Could you check a few things on this model? Use its own coordinates, in mm. A direction names the side the tool comes from. Coordinates: 2 decimals unless noted, no trailing zeros. Write each loop counter-clockwise with the first axis right and the second up, starting at its lowest first coordinate (ties: lowest second). Pieces come first, ordered by that corner, then holes.
Item 1: If I drill on probe 1 along Y at (x, z) = (2, -11.5); probe 2 along X at (y, z) = (45, -7.25); probe 3 along Y at (x, z) = (3, -6.5), over which ranges is the centre line in solid material (lowest first)?
Item 2: I want a section at C-C on x = 13. Please give me the cut outline in (y, z).
Item 3: I want a section at B-B on y = 51.5. Please give me the cut outline in (x, z).
Item 4: Which directions (+Z, -Z, +X, -X, +Y, -Y) give clear straight access to the entire face, cutting with the end or side of a thin tool? Please do faces 5 (the flat face through (9, 153.67, -4)), 6 (the flat face through (1, 0, -2)), 7 (the flat face through (-11, 0, -12)).
Item 5: I want a section at A-A on x = -9.5. Please give me the cut outline in (y, z).
Item 6: For P1, Ø1.5, axis at x = 4.5, y = 38, coming from the -Z side; P2, Ø0.6, axis at x = 1.5, z = -11.5, coming from the -Y side; P3, Ø1, axis at y = 22, z = -2.5, coming from the -X side; P4, Ø1.5, axis at y = 115.5, z = -6, coming from the +X side, each with a flat end and sliding along its axis, tell me the tip position at first contact or that it passes through.
Item 7: Thinking about a two-plate mould opening in X: for faces 1 (the flat face through (2.172, 77, -4)), 2 (the flat face through (9, 152.4, -4)), 3 (the flat face through (-0.876, 76, -4)), 4 (the flat face through (1, 0, -7)), which applies, +X half, -X half, draft (parallel to the pull), parting line (faces both ways), or undercut?
from build123d import *

# Parameters (mm, degrees)
BOSS_EXTRUDE1_DEPTH = 152.4
SKETCH2_W           = 19.05
SKETCH2_H           = 19.05
BOSS_EXTRUDE2_DEPTH = 1.27
SKETCH3_R           = 1.016
BOSS_EXTRUDE3_DEPTH = 8.89
BOSS_EXTRUDE4_DEPTH = 1.27
SKETCH5_W           = 15.24
SKETCH5_H           = 12.7
CUT_EXTRUDE1_DEPTH  = 2.27


with BuildPart() as part:
    # Sketch1 → Boss-Extrude1 (new body)
    with BuildSketch(Plane(origin=(0, 0, 0), x_dir=(1, 0, 0), z_dir=(0, 1, 0))):
        Polygon((0.1397, 7.023481), (-0.8763, 7.023481), (-0.8763, 1.305306), (0.1397, 1.305306), (0.1397, 0), (2.1717, 0), (2.1717, 8.328787), (0.1397, 8.328787), align=None)
    extrude(amount=BOSS_EXTRUDE1_DEPTH)

    # Sketch2 → Boss-Extrude2 (add)
    with BuildSketch(Plane(origin=(0, 152.4, 0), x_dir=(1, 0, 0), z_dir=(0, 1, 0))):
        with Locations((8.6487, 4.1643935)):
            Rectangle(SKETCH2_W, SKETCH2_H)
    extrude(amount=BOSS_EXTRUDE2_DEPTH)

    # Sketch3 → Boss-Extrude3 (add)
    with BuildSketch(Plane.XZ.offset(-152.4)):
        with Locations((15.602834065, 2.789740565)):
            Circle(SKETCH3_R)
        with Locations((15.602834065, -11.118527565)):
            Circle(SKETCH3_R)
        with Locations((1.694565935, -11.118527565)):
            Circle(SKETCH3_R)
        with Locations((1.694565935, 2.789740565)):
            Circle(SKETCH3_R)
    extrude(amount=BOSS_EXTRUDE3_DEPTH)

    # Sketch4 → Boss-Extrude4 (add)
    with BuildSketch(Plane.XZ):
        Polygon((-21.9583, 4.8356065), (-1.6383, 4.8356065), (-1.6383, -3.5293935), (2.1717, -3.5293935), (2.1717, -4.7993935), (-1.6383, -4.7993935), (-1.6383, -13.1643935), (-21.9583, -13.1643935), align=None)
    extrude(amount=BOSS_EXTRUDE4_DEPTH)

    # Sketch5 → Cut-Extrude1 (cut, through all)
    with BuildSketch(Plane(origin=(0, 0, 0), x_dir=(1, 0, 0), z_dir=(0, 1, 0))):
        with Locations((-11.7983, 4.1643935)):
            Rectangle(SKETCH5_W, SKETCH5_H)
    extrude(amount=-CUT_EXTRUDE1_DEPTH, mode=Mode.SUBTRACT)


solid = part.part
Response values:
1. probe 1: y = 143.51 to 153.67
1. probe 2: x = 0.14 to 2.17
1. probe 3: y = 152.4 to 153.67
2. outline: (152.4, -13.69) - (153.67, -13.69) - (153.67, 5.36) - (152.4, 5.36) - close
3. outline: (-0.88, -7.02) - (0.14, -7.02) - (0.14, -8.33) - (2.17, -8.33) - (2.17, 0) - (0.14, 0) - (0.14, -1.31) - (-0.88, -1.31) - close
4. face 5: +Z, -Z, +X, -X, +Y
4. face 6: +Z, +X, -Y
4. face 7: +Z, -Z, -X, +Y
5. outline: (-1.27, -13.16) - (0, -13.16) - (0, -10.51) - (-1.27, -10.51) - close; (-1.27, 2.19) - (0, 2.19) - (0, 4.84) - (-1.27, 4.84) - close
6. P1: passes through
6. P2: stops at y = 143.51
6. P3: stops at x = -0.88
6. P4: stops at x = 2.17
7. face 1: +X half
7. face 2: undercut
7. face 3: -X half
7. face 4: draft
